```python
from build123d import *

# Parameters (mm, degrees)
F0_W     = 101.6
F0_H     = 50.8
F1_DEPTH = 25.4
F2_R     = 6.35
F3_DEPTH = 25.401
F4_W     = 12.7
F4_H     = 25.4
F6_W     = 10.16
F6_H     = 6.35
F8_R     = 1.27
F9_SIZE  = 2.54


with BuildPart() as f1:
    # F0 (on Front) → F1 (new body)
    with BuildSketch(Plane.XZ):
        Rectangle(F0_W, F0_H)
    extrude(amount=F1_DEPTH)

    # F2 (on face) → F3 (cut, through all)
    with BuildSketch(Plane.XZ.offset(25.4)):
        with Locations((-38.1, 12.7)):
            Circle(F2_R)
        with Locations((-38.1, -12.7)):
            Circle(F2_R)
        with Locations((38.1, 12.7)):
            Circle(F2_R)
        with Locations((38.1, -12.7)):
            Circle(F2_R)
    extrude(amount=-F3_DEPTH, mode=Mode.SUBTRACT)

    # F4 (on Top) → F5 (revolve)
    with BuildSketch(Plane.XY):
        with Locations((6.35, -38.1)):
            Rectangle(F4_W, F4_H)
    revolve(axis=Axis((0, -38.1, 0), (0, 1, 0)))

    # F6 (on Top) → F7 (revolve, cut)
    with BuildSketch(Plane.XY):
        with Locations((11.866805, -38.735)):
            Rectangle(F6_W, F6_H)
    revolve(axis=Axis((0, -36.219459, 0), (0, -1, 0)), mode=Mode.SUBTRACT)

    # F8
    f8_edges = [f1.edges().sort_by_distance(p)[0] for p in [
        (-12.7, -25.4, 0),
        (-6.786805, -41.91, 0),
        (-6.786805, -35.56, 0),
    ]]
    fillet(f8_edges, radius=F8_R)

    # F9
    f9_edges = [f1.edges().sort_by_distance(p)[0] for p in [
        (0, -25.4, -25.4),
        (0, -25.4, 25.4),
        (-50.8, -25.4, 0),
        (50.8, -25.4, 0),
    ]]
    chamfer(f9_edges, length=F9_SIZE)


solid = f1.part
```
Design review of the part built by this model. Coordinates are the model's own, in mm. A direction names the side the tool comes from. Give positions to 0.01 mm unless a question says otherwise; leave off trailing zeros. Order: outer loops, then holes, each group sorted by start corner. A loop starts at its lowest first (then second) coordinate and runs counter-clockwise, first axis right, second up. Notation, with made-up numbers: (69.25, 57.25) -> (126.25, 57.25) arc R26 cw to (126.25, 83.25) -> close; hole circle Ø3 at (41, 84). An arc over 180 degrees is marked (long way). Write each question's results on one line, items separated by ' | '. Start each with the question number.
Q1. Wall thickness on L1, parallel to Z at x = -38, y = -14; L2, parallel to X at y = -13.5, z = -7.5; L3, parallel to X at y = -11, z = 11: over which ranges is each line inside the solid? List them lowest first. Write a range as from..to.
Q2. Machinability: for faces 1 (the flat face through (0.2, -35.56, -8.3)), 2 (the flat face through (-49.55, -24.11, -0.36)), 3 (the cylindrical face through (-2.75, -31.05, 12.4)), which of the approach directions +Z, -Z, +X, -X, +Y, -Y give a long, thin tool a straight path to every point of the face, cutting with its end or side? Answer none if there is none.
Q3. Add section C-C on y = -4. Give the boundary of the cut face in (x, z), and give its area (3 significant figures).
Q4. Add section B-B on z = 16.5. Give the boundary of the cut face in (x, y), and give its area (3 significant figures).
Q5. Add section D-D on x = 0. Give the boundary of the cut face in (y, z).
Q6. For pin 1 (6 mm diameter, centred on x = 19, z = -16, fed in from +Y); pin 2 (6 mm diameter, centred on x = 33, z = -3, fed in from -Y), all flat-tipped, find the tip position at first contact; note any pin that passes through.
Q7. Add section A-A on x = 38.1. Give the boundary of the cut face in (y, z).
Q8. Mouldability with a two-part tool opening along Z and no side actions: class faces 4 (the cylindrical face through (31.756, -12.878, 12.979)), 5 (the flat face through (0, -50.8, 0)), 6 (the cylindrical face through (-2.75, -46.29, 12.4)) as +Z half, -Z half, draft (parallel to the pull), parting line (faces both ways), or undercut.
Found:
1) L1: z = -25.4..-19.05, -6.35..6.35, 19.05..25.4 | L2: x = -50.8..-41.74, -34.46..34.46, 41.74..50.8 | L3: x = -50.8..-44.22, -31.98..31.98, 44.22..50.8
2) face 1: none | face 2: +Z, -Z, -X, -Y | face 3: -Y
3) outline: (-50.8, -25.4) -> (50.8, -25.4) -> (50.8, 25.4) -> (-50.8, 25.4) -> close; hole circle Ø12.7 at (-38.1, -12.7); hole circle Ø12.7 at (-38.1, 12.7); hole circle Ø12.7 at (38.1, -12.7); hole circle Ø12.7 at (38.1, 12.7) | area: 4,650 mm2
4) outline: (-50.8, -22.86) -> (-48.26, -25.4) -> (-43.19, -25.4) -> (-43.19, 0) -> (-50.8, 0) -> close; (-33.01, -25.4) -> (33.01, -25.4) -> (33.01, 0) -> (-33.01, 0) -> close; (43.19, -25.4) -> (48.26, -25.4) -> (50.8, -22.86) -> (50.8, 0) -> (43.19, 0) -> close | area: 2,060 mm2
5) outline: (-50.8, -12.7) -> (-41.91, -12.7) -> (-41.91, -8.06) arc R1.27 cw to (-40.64, -6.79) -> (-36.83, -6.79) arc R1.27 cw to (-35.56, -8.06) -> (-35.56, -12.7) -> (-26.67, -12.7) arc R1.27 cw to (-25.4, -13.97) -> (-25.4, -22.86) -> (-22.86, -25.4) -> (0, -25.4) -> (0, 25.4) -> (-22.86, 25.4) -> (-25.4, 22.86) -> (-25.4, 13.97) arc R1.27 cw to (-26.67, 12.7) -> (-35.56, 12.7) -> (-35.56, 8.06) arc R1.27 cw to (-36.83, 6.79) -> (-40.64, 6.79) arc R1.27 cw to (-41.91, 8.06) -> (-41.91, 12.7) -> (-50.8, 12.7) -> close
6) pin 1: stops at y = 0 | pin 2: stops at y = -25.4
7) outline: (-25.4, -22.86) -> (-22.86, -25.4) -> (0, -25.4) -> (0, -19.05) -> (-25.4, -19.05) -> close; (-25.4, -6.35) -> (0, -6.35) -> (0, 6.35) -> (-25.4, 6.35) -> close; (-25.4, 19.05) -> (0, 19.05) -> (0, 25.4) -> (-22.86, 25.4) -> (-25.4, 22.86) -> close
8) face 4: undercut | face 5: draft | face 6: parting line
